Read the model definition and answer for the solid it produces. Units are mm, in the model's axes. A direction names the side the tool comes from. Round coordinates to 2 decimals unless told otherwise and drop trailing zeros. Loops run counter-clockwise (first coordinate to the right, second up) from the corner with the lowest first, then second, coordinate; pieces in that order, holes last. Notation, with made-up numbers: (8.5, -12) - (33.5, -12) arc R32 cw to (33.5, 18) - close; hole circle Ø10 at (-36, -31). An arc over 180 degrees is marked (long way). Use one line per item in the form item = value. Start each with the question number.
```python
from build123d import *

# Parameters (mm, degrees)
EXTRUDE_THIN1_DEPTH = 25
SKETCH2_R           = 5.5
CUT_EXTRUDE1_DEPTH  = 5


with BuildPart() as part:
    # Sketch1 → Extrude-Thin1 (new, symmetric)
    with BuildSketch(Plane.XY):
        Polygon((50, 0), (0, 0), (0, 50), (5, 50), (5, 5), (50, 5), align=None)
    extrude(amount=EXTRUDE_THIN1_DEPTH, both=True)

    # Sketch2 → Cut-Extrude1 (cut)
    with BuildSketch(Plane.YZ):
        with Locations(Location((25, 0, 0), (0, 0, 270))):
            Circle(SKETCH2_R)
    extrude(amount=CUT_EXTRUDE1_DEPTH, mode=Mode.SUBTRACT)


solid = part.part
```
1) A cutting plane is placed at C-C on z = 17. Write down the section's boundary in (x, y), plus the area to 3 significant figures.
2) A cutting plane is placed at A-A on y = 25. Write down the section's boundary in (x, z), plus the area to 3 significant figures.
3) A cutting plane is placed at B-B on z = 0. Write down the section's boundary in (x, y), plus the area to 3 significant figures.
4) A cutting plane is placed at D-D on y = 46.5. Write down the section's boundary in (x, z), plus the area to 3 significant figures.
5) Straight lines are drawn through the part: line 1 (Y direction, x = 1.2, z = 0); line 2 (Y direction, x = 31, z = -10). For each, find the intervals that lie inside material, in ascending order. Write a range as from..to.
6) Flat-ended cylindrical pins translate along their axes: pin 1 (22.5 mm diameter, centred on y = 26.5, z = -6.5, fed in from +X); pin 2 (4 mm diameter, centred on y = 20.5, z = -1.5, fed in from -X). Find the tip coordinate at first contact, or state that the pin passes through.
7) For faces 1 (the cylindrical face through (2.465, 30.453, 0.716)), 2 (the flat face through (27, 5, 0)), determine the directions among +Z, -Z, +X, -X, +Y, -Y from which every point of the face is accessible in a straight line to the end or side of a thin tool.
Checks:
q1.outline = (0, 0) - (50, 0) - (50, 5) - (5, 5) - (5, 50) - (0, 50) - close
q1.area = 475 mm²
q2.outline = (0, -25) - (5, -25) - (5, -5.5) - (0, -5.5) - close; (0, 5.5) - (5, 5.5) - (5, 25) - (0, 25) - close
q2.area = 195 mm²
q3.outline = (0, 0) - (50, 0) - (50, 5) - (5, 5) - (5, 19.5) - (0, 19.5) - close; (0, 30.5) - (5, 30.5) - (5, 50) - (0, 50) - close
q3.area = 420 mm²
q4.outline = (0, -25) - (5, -25) - (5, 25) - (0, 25) - close
q4.area = 250 mm²
q5.line_1 = 0..19.5, 30.5..50
q5.line_2 = 0..5
q6.pin_1 = 5
q6.pin_2 = 0
q7.face_1 = +X, -X
q7.face_2 = +Z, -Z, +X, +Y
